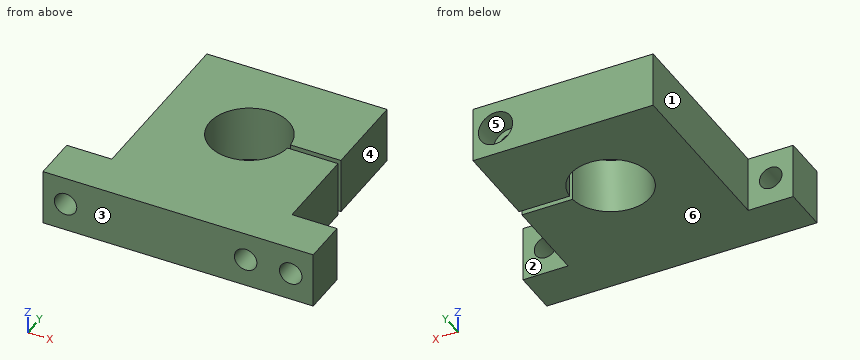
Autodesk Inventor part; units mm, degrees
ref_plane "YZ Plane" through (0, 0, 0) normal (1, 0, 0) x (0, 1, 0)
ref_plane "XZ Plane" through (0, 0, 0) normal (0, 1, 0) x (-1, 0, 0)
ref_plane "XY Plane" through (0, 0, 0) normal (0, 0, 1) x (1, 0, 0)
sketch "Sketch1" plane through (0, 0, 0) normal (0, 0, 1) x (1, 0, 0)
  line L0 (0, 0) -> (76.2, 0)
  line L1 (76.2, 0) -> (76.2, 12.7)
  line L2 (76.2, 12.7) -> (63.5, 12.7)
  line L3 (63.5, 12.7) -> (63.5, 63.5)
  line L4 (63.5, 63.5) -> (12.7, 63.5)
  line L5 (12.7, 63.5) -> (12.7, 12.7)
  line L6 (12.7, 12.7) -> (0, 12.7)
  line L7 (0, 12.7) -> (0, 0)
  dimension "d0" = 12.7
  dimension "d1" = 12.7
  dimension "d2" = 76.2
  dimension "d3" = 50.8
  dimension "d4" = 12.7
extrude "Extrusion1" add sketch "Sketch1" along normal blind 15.748
sketch "Sketch2" plane through (0, 0, 15.748) normal (0, 0, 1) x (1, 0, 0)
  arc A0 (49.25, 38.862) -> (49.25, 37.338) centre (38.1, 38.1) ccw
  line L0 (12.7, 63.5) -> (12.7, 12.7)
  line L1 (63.5, 63.5) -> (12.7, 63.5)
  line L2 (63.5, 38.862) -> (49.25, 38.862)
  line L3 (49.25, 37.338) -> (63.5, 37.338)
  line L4 (63.5, 12.7) -> (63.5, 63.5)
  line L5 (63.5, 38.862) -> (63.5, 37.338)
  point P0 (0, 0)
  dimension "d7" = 22.352
  dimension "d8" = 25.4
  dimension "d9" = 25.4
  dimension "d10" = 1.524
  dimension "d11" = 24.638
extrude "Extrusion2" cut sketch "Sketch2" against normal blind 15.748
sketch "Sketch3" plane through (63.5, 12.7, 0) normal (0, 1, 0) x (1, 0, 0)
  line L0 (-50.8, -15.748) -> (-63.5, -15.748)
  line L1 (-63.5, 0) -> (-63.5, -15.748)
  line L2 (12.7, 0) -> (12.7, -15.748)
  line L3 (12.7, -15.748) -> (0, -15.748)
  point P0 (-57.15, -7.874)
  point P1 (6.35, -7.874)
  dimension "d14" = 7.874
  dimension "d15" = 6.35
  dimension "d16" = 6.35
  dimension "d17" = 7.874
hole "Hole1" at (6.35, 12.7, 7.874) at (69.85, 12.7, 7.874) direction (0, -1, 0) diameter 6.35 end through all
sketch "Sketch4" plane through (12.7, 63.5, 0) normal (0, 1, 0) x (1, 0, 0)
  line L0 (50.8, 0) -> (0, 0)
  line L1 (50.8, 0) -> (50.8, -15.748)
  point P0 (-12.7, 0)
  point P1 (44.45, -7.874)
  dimension "d25" = 7.874
  dimension "d26" = 6.35
hole "Hole2" at (57.15, 63.5, 7.874) direction (0, -1, 0) diameter 6.35 end through all counterbore diameter 9.652 counterbore depth 7.874
properties part number "Figure 6_16_W"
Verification items for the finished model (mm, model axes). Face numbers are marked on the shaded views. A direction names the side the tool comes from. Round coordinates to 2 decimals unless told otherwise and drop trailing zeros. Order: outer loops, then holes, each group sorted by start corner. A loop starts at its lowest first (then second) coordinate and runs counter-clockwise, first axis right, second up.
1. Access from +Z, -Z, +X, -X, +Y, -Y to the whole of each face (thin tool, end or side, straight path). Record for the marked faces 1, 2 and 3.
Final values:
face 1: +Z, -Z, -X, +Y
face 2: +Z, -Z, +X, +Y
face 3: +Z, -Z, +X, -X, -Y
2. Go/stop test with flat-tipped pins: P1, Ø8, axis at y = 35.5, z = 13, coming from the -X side; P2, Ø7.5, axis at x = 6.35, z = 7.874, coming from the +Y side; P3, Ø4.5, axis at y = 50, z = 4, coming from the +X side; P4, Ø5.5, axis at x = 57.15, z = 7.874, coming from the +Y side. Record where each tip stops, or that it passes through.
Final values:
P1: stops at x = 12.7
P2: stops at y = 12.7
P3: stops at x = 63.5
P4: passes through
3. Section check B-B on y = 4.5. Record the cut outline in (x, z) (3 decimals).
Final values:
outline: (0, 0) - (76.2, 0) - (76.2, 15.748) - (0, 15.748) - close; hole circle Ø6.35 at (6.35, 7.874); hole circle Ø6.35 at (57.15, 7.874); hole circle Ø6.35 at (69.85, 7.874)
4. Section check C-C on x = 38.1. Record the cut outline in (y, z), then the cut area to 3 significant figures.
Final values:
outline: (0, 0) - (26.92, 0) - (26.92, 15.75) - (0, 15.75) - close; (49.28, 0) - (63.5, 0) - (63.5, 15.75) - (49.28, 15.75) - close
area: 648 mm2
5. Section check D-D on z = 9.25. State how many separate pieces and enclosed holes the cut face has, then the cut area to 3 significant figures.
Final values:
separate pieces: 5
enclosed holes: 0
area: 2,610 mm2
6. Thickness scan on L1, parallel to Z at x = 6.35, y = 9; L2, parallel to Y at x = 38.1, z = 5.75; L3, parallel to X at y = 5.5, z = 6. Record the ranges inside material, lowest first.
Final values:
L1: z = 0 to 4.7, 11.05 to 15.75
L2: y = 0 to 26.92, 49.28 to 63.5
L3: x = 0 to 3.79, 8.91 to 54.59, 59.71 to 67.29, 72.41 to 76.2
7. Section check A-A on x = 57.15. Record the cut outline in (y, z).
Final values:
outline: (0, 0) - (37.34, 0) - (37.34, 4.7) - (0, 4.7) - close; (0, 11.05) - (37.34, 11.05) - (37.34, 15.75) - (0, 15.75) - close; (38.86, 0) - (63.5, 0) - (63.5, 3.05) - (55.63, 3.05) - (55.63, 4.7) - (38.86, 4.7) - close; (38.86, 11.05) - (55.63, 11.05) - (55.63, 12.7) - (63.5, 12.7) - (63.5, 15.75) - (38.86, 15.75) - close
8. Release check for a two-part mould opening along X. For the marked faces 4, 5 and 6 record: +X half, -X half, draft (parallel to the pull), parting line (faces both ways), or undercut.
Final values:
face 4: +X half
face 5: undercut
face 6: draft
